Input: part model. Units: mm. Frame: model coordinates. Face numbers are marked on the shaded views. Coordinates: 2 decimals unless noted, no trailing zeros. Write each loop counter-clockwise with the first axis right and the second up, starting at its lowest first coordinate (ties: lowest second). Pieces come first, ordered by that corner, then holes. Notation, with made-up numbers: M 35,-26.75 L 80,-26.75 A8 cw 80,-22.75 Z; hole C 21,29 d5. An arc over 180 degrees is marked long. Answer as a JSON object with one key per item and string values. Group by question number.
from build123d import *

# Parameters (mm, degrees)
SKETCH2_W           = 4.86
SKETCH2_H           = 1.78
BOSS_EXTRUDE1_DEPTH = 4.6
SKETCH3_R           = 0.22
CUT_EXTRUDE1_DEPTH  = 4.5
SKETCH4_W           = 0.2
SKETCH4_H           = 0.06
BOSS_EXTRUDE2_DEPTH = 1.96
SKETCH6_W           = 0.2
SKETCH6_H           = 0.06
BOSS_EXTRUDE3_DEPTH = 0.69
SKETCH7_W           = 0.2
SKETCH7_H           = 0.06
BOSS_EXTRUDE4_DEPTH = 1.7
SKETCH8_W           = 0.2
SKETCH8_H           = 0.06
BOSS_EXTRUDE5_DEPTH = 2.46


with BuildPart() as part:
    # Sketch2 → Boss-Extrude1 (new body)
    with BuildSketch(Plane(origin=(0, 0, 0), x_dir=(1, 0, 0), z_dir=(0, 1, 0))):
        with Locations((2.43, 0.89)):
            Rectangle(SKETCH2_W, SKETCH2_H)
    extrude(amount=BOSS_EXTRUDE1_DEPTH)

    # Sketch3 → Cut-Extrude1 (cut)
    with BuildSketch(Plane(origin=(0, 4.6, 0), x_dir=(1, 0, 0), z_dir=(0, 1, 0))):
        with Locations((0.51, 1.27)):
            Circle(SKETCH3_R)
        with Locations((1.15, 1.27)):
            Circle(SKETCH3_R)
        with Locations((1.79, 1.27)):
            Circle(SKETCH3_R)
        with Locations((2.43, 1.27)):
            Circle(SKETCH3_R)
        with Locations((3.07, 1.27)):
            Circle(SKETCH3_R)
        with Locations((3.71, 1.27)):
            Circle(SKETCH3_R)
        with Locations((4.35, 1.27)):
            Circle(SKETCH3_R)
        with Locations((1.15, 0.51)):
            Circle(SKETCH3_R)
        with Locations((1.79, 0.51)):
            Circle(SKETCH3_R)
        with Locations((2.43, 0.51)):
            Circle(SKETCH3_R)
        with Locations((3.07, 0.51)):
            Circle(SKETCH3_R)
        with Locations((3.71, 0.51)):
            Circle(SKETCH3_R)
        with Locations((4.35, 0.51)):
            Circle(SKETCH3_R)
        with Locations((0.51, 0.51)):
            Circle(SKETCH3_R)
    extrude(amount=-CUT_EXTRUDE1_DEPTH, mode=Mode.SUBTRACT)

    # Sketch4 → Boss-Extrude2 (add)
    with BuildSketch(Plane.XZ):
        with Locations((0.51, -0.51)):
            Rectangle(SKETCH4_W, SKETCH4_H)
        with Locations((1.15, -0.51)):
            Rectangle(SKETCH4_W, SKETCH4_H)
        with Locations((1.79, -0.51)):
            Rectangle(SKETCH4_W, SKETCH4_H)
        with Locations((2.43, -0.51)):
            Rectangle(SKETCH4_W, SKETCH4_H)
        with Locations((3.07, -0.51)):
            Rectangle(SKETCH4_W, SKETCH4_H)
        with Locations((3.71, -0.51)):
            Rectangle(SKETCH4_W, SKETCH4_H)
        with Locations((4.35, -0.51)):
            Rectangle(SKETCH4_W, SKETCH4_H)
    extrude(amount=BOSS_EXTRUDE2_DEPTH)

    # Sketch6 → Boss-Extrude3 (add)
    with BuildSketch(Plane.XZ):
        with Locations((0.51, -1.27)):
            Rectangle(SKETCH6_W, SKETCH6_H)
        with Locations((1.15, -1.27)):
            Rectangle(SKETCH6_W, SKETCH6_H)
        with Locations((1.79, -1.27)):
            Rectangle(SKETCH6_W, SKETCH6_H)
        with Locations((2.43, -1.27)):
            Rectangle(SKETCH6_W, SKETCH6_H)
        with Locations((3.07, -1.27)):
            Rectangle(SKETCH6_W, SKETCH6_H)
        with Locations((3.71, -1.27)):
            Rectangle(SKETCH6_W, SKETCH6_H)
        with Locations((4.35, -1.27)):
            Rectangle(SKETCH6_W, SKETCH6_H)
    extrude(amount=BOSS_EXTRUDE3_DEPTH)

    # Sketch7 → Boss-Extrude4 (add)
    with BuildSketch(Plane(origin=(0, 0, -1.3), x_dir=(-1, 0, 0), z_dir=(0, 0, -1))):
        with Locations((-4.35, -0.66)):
            Rectangle(SKETCH7_W, SKETCH7_H)
        with Locations((-3.71, -0.66)):
            Rectangle(SKETCH7_W, SKETCH7_H)
        with Locations((-3.07, -0.66)):
            Rectangle(SKETCH7_W, SKETCH7_H)
        with Locations((-2.43, -0.66)):
            Rectangle(SKETCH7_W, SKETCH7_H)
        with Locations((-1.79, -0.66)):
            Rectangle(SKETCH7_W, SKETCH7_H)
        with Locations((-1.15, -0.66)):
            Rectangle(SKETCH7_W, SKETCH7_H)
        with Locations((-0.51, -0.66)):
            Rectangle(SKETCH7_W, SKETCH7_H)
    extrude(amount=BOSS_EXTRUDE4_DEPTH)

    # Sketch8 → Boss-Extrude5 (add)
    with BuildSketch(Plane(origin=(0, 0, -0.54), x_dir=(-1, 0, 0), z_dir=(0, 0, -1))):
        with Locations((-4.35, -1.93)):
            Rectangle(SKETCH8_W, SKETCH8_H)
        with Locations((-3.71, -1.93)):
            Rectangle(SKETCH8_W, SKETCH8_H)
        with Locations((-3.07, -1.93)):
            Rectangle(SKETCH8_W, SKETCH8_H)
        with Locations((-2.43, -1.93)):
            Rectangle(SKETCH8_W, SKETCH8_H)
        with Locations((-1.79, -1.93)):
            Rectangle(SKETCH8_W, SKETCH8_H)
        with Locations((-1.15, -1.93)):
            Rectangle(SKETCH8_W, SKETCH8_H)
        with Locations((-0.51, -1.93)):
            Rectangle(SKETCH8_W, SKETCH8_H)
    extrude(amount=BOSS_EXTRUDE5_DEPTH)


solid = part.part
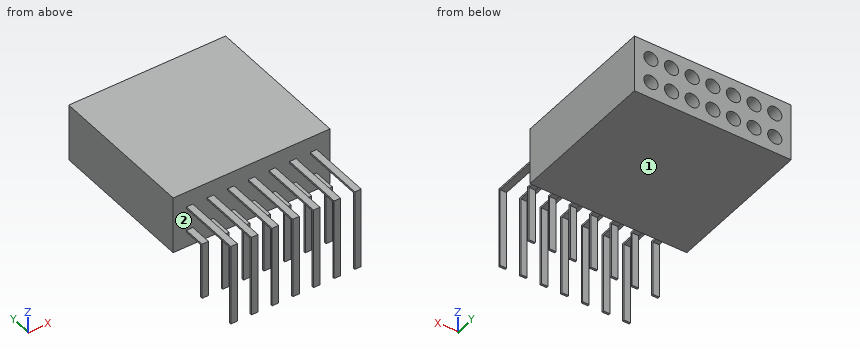
Q1. Section A-A, the plane y = 1.5. State how many separate pieces and enclosed holes the cut face has, and give its area (3 significant figures).
Q2. Section D-D, the plane x = 1.79. Return the cut outline in (y, z).
Q3. Line query: line 1 (Z direction, x = 3.1, y = 4); line 2 (Y direction, x = 0.2, z = -0.8); line 3 (Z direction, x = 4, y = 3). Output: solid intervals per line, ascending. Write a range as from..to.
Q4. Pin query (flat end, axial travel): pin 1 Ø1 at (x, y) = (1.5, 3.5) entering from +Z; pin 2 Ø1 at (x, y) = (3, 3.5) entering from -Z. Return the tip coordinate at first contact, or that it passes through.
Q5. Draft query along Y for the marked faces 1 and 2. Return one class per face: released by +Y, released by -Y, zero draft, split by the parting line, or undercut.
Filled in:
{
 "1": {"separate pieces": "1", "enclosed holes": "14", "area": "6.52 mm^2"},
 "2": {"outline": "M -1.96,-3 L -1.9,-3 L -1.9,-0.54 L 0,-0.54 L 0,-1.24 L -0.69,-1.24 L -0.69,-3 L -0.63,-3 L -0.63,-1.3 L 0,-1.3 L 0,-1.78 L 4.6,-1.78 L 4.6,-1.49 L 0.1,-1.49 L 0.1,-1.05 L 4.6,-1.05 L 4.6,-0.73 L 0.1,-0.73 L 0.1,-0.29 L 4.6,-0.29 L 4.6,0 L 0,0 L 0,-0.48 L -1.96,-0.48 Z"},
 "3": {"line 1": "-1.78..-1.49, -1.05..-0.73, -0.29..0", "line 2": "0..4.6", "line 3": "-1.78..0"},
 "4": {"pin 1": "z = 0", "pin 2": "z = -1.78"},
 "5": {"face 1": "zero draft", "face 2": "undercut"}
}
